CAD build for the part. Positions are in the model's coordinates, mm. A direction names the side the tool comes from. Round coordinates to 2 decimals unless told otherwise and drop trailing zeros. Write each loop counter-clockwise with the first axis right and the second up, starting at its lowest first coordinate (ties: lowest second). Pieces come first, ordered by that corner, then holes. Notation, with made-up numbers: (23.25, 46.5) -> (66.25, 46.5) arc R19 ccw to (66.25, 74.5) -> close; hole circle Ø3 at (-31.5, -14). An arc over 180 degrees is marked (long way). Put each result on its own line as item: value. Start each with the question number.
1. 3-axis set-ups, long thin cutter, end or side, ignore diameter. For faces 4 (the cylindrical face through (5, -15, -28)), 5 (the flat face through (5, -18, -26)), 6 (the flat face through (1, -15, 29)): which of +Z, -Z, +X, -X, +Y, -Y reach the whole face in a straight line?
2. Flat gauge pins, fed straight in: P1, Ø3, axis at x = 3, y = -17, coming from the +Z side; P2, Ø4, axis at x = 5, z = 32.5, coming from the +Y side; P3, Ø0.7, axis at x = 8.5, y = -15.5, coming from the -Z side. Where does each tip first touch, or does it go through?
3. Drill centre lines: line 1 (Z direction, x = 5, y = -32.75); line 2 (Z direction, x = 0.75, y = -6.5); line 3 (X direction, y = -33.7, z = -32.5). Where is each one in solid material? Low to high. Write a range as from..to.
4. Saw through at D-D on z = 20.5. List the corners of the cut face in (x, y).
5. Saw through at C-C on x = 1. List the corners of the cut face in (y, z).
6. Saw through at A-A on x = 5. List the corners of the cut face in (y, z).
7. Pull direction Z, two halves, no side cores. Call faces 1 (the cylindrical face through (5, -15, 28)), 2 (the flat face through (4.9, -35, 30.6)), 3 (the cylindrical face through (5.07, -0.57, 25.4)): pulls with the +Z half, pulls with the -Z half, needs draft (parallel to the pull), parting line crosses it, or undercut.
8. Saw through at B-B on z = 32.5. List the corners of the cut face in (x, y).
Autodesk Inventor part; units mm, degrees
ref_plane "YZ Plane" through (0, 0, 0) normal (1, 0, 0) x (0, 1, 0)
ref_plane "XZ Plane" through (0, 0, 0) normal (0, 1, 0) x (-1, 0, 0)
ref_plane "XY Plane" through (0, 0, 0) normal (0, 0, 1) x (1, 0, 0)
sketch "Sketch1" plane through (0, 0, 0) normal (1, 0, 0) x (0, 1, 0)
  line L0 (0, 0) -> (0, 26)
  line L1 (0, 26) -> (-35, 26)
  line L2 (0, 0) -> (3, 0)
  line L3 (3, 0) -> (3, 29)
  line L4 (3, 29) -> (-32, 29)
  line L5 (-32, 29) -> (-32, 36)
  line L6 (-32, 36) -> (-35, 36)
  line L7 (-35, 36) -> (-35, 26)
  line L8 (0, 0) -> (0, -26)
  line L9 (0, -26) -> (-35, -26)
  line L10 (3, 0) -> (3, -29)
  line L11 (3, -29) -> (-32, -29)
  line L12 (-32, -29) -> (-32, -36)
  line L13 (-32, -36) -> (-35, -36)
  line L14 (-35, -36) -> (-35, -26)
  dimension "d0" = 26
  dimension "d1" = 35
  dimension "d2" = 3
  dimension "d3" = 29
  dimension "d4" = 35
  dimension "d5" = 7
extrude "Extrusion1" add sketch "Sketch1" along normal blind 10
fillet "Fillet1" radius 2 4 edges at (5, 3, 29) (5, 0, 26) (5, 0, -26) (5, 3, -29)
sketch "Sketch2" plane through (0, -32, 36) normal (0, 1, 0) x (1, 0, 0)
  line L0 (0, 7) -> (0, 0)
  line L1 (0, 3.5) -> (5, 3.5)
  line L2 (0, 62) -> (0, 72)
  line L3 (0, 72) -> (0, 68.5)
  line L4 (0, 68.5) -> (5, 68.5)
  point P0 (0, 36)
  dimension "d9" = 3.5
hole "Hole1" at (5, -32, 32.5) at (5, -32, -32.5) direction (0, -1, 0) diameter 3.4 end through all
sketch "Sketch3" plane through (0, -32, 36) normal (0, 1, 0) x (1, 0, 0)
  circle A0 centre (5, 3.5) radius 1.7
  circle A1 centre (5, 3.5) radius 4.5
  circle A2 centre (5, 68.5) radius 1.7
  circle A3 centre (5, 68.5) radius 4.5
  point P0 (0, 36)
  dimension "d17" = 9
  dimension "d18" = 9
extrude "Extrusion2" cut sketch "Sketch3" along normal through all
sketch "Sketch4" plane through (0, -35, 36) normal (0, 0, 1) x (1, 0, 0)
  line L0 (0, 3) -> (2.1716, 3)
  line L1 (0, 0) -> (10, 0)
  line L2 (0, 3) -> (10, 3)
  line L3 (10, 3) -> (10, 0)
  line L4 (10, 0) -> (0, 0)
  line L5 (0, 0) -> (0, 3)
  point P0 (0, 35)
extrude "Extrusion3" add sketch "Sketch4" along normal blind 2
sketch "Sketch5" plane through (0, -35, -36) normal (0, 0, -1) x (-1, 0, 0)
  line L0 (0, 0) -> (-10, 0)
  line L1 (0, 3) -> (-10, 3)
  line L2 (-10, 3) -> (-10, 0)
  line L3 (-10, 0) -> (0, 0)
  line L4 (0, 0) -> (0, 3)
  point P0 (0, 35)
extrude "Extrusion4" add sketch "Sketch5" along normal blind 2
properties part number "battery-bracket"
Return value:
1. face 4: -Z, +Y
1. face 5: +X, -X, -Y
1. face 6: +Z, +X, -X, +Y
2. P1: stops at z = 29
2. P2: stops at y = -32
2. P3: stops at z = -29
3. line 1: z = -38..-34.2, -30.8..-26, 26..30.8, 34.2..38
3. line 2: z = -29..-26, 26..29
3. line 3: x = 0..3.3, 6.7..10
4. outline: (0, 0) -> (10, 0) -> (10, 3) -> (0, 3) -> close
5. outline: (-35, -38) -> (-32, -38) -> (-32, -29) -> (1, -29) arc R2 ccw to (3, -27) -> (3, 27) arc R2 ccw to (1, 29) -> (-32, 29) -> (-32, 38) -> (-35, 38) -> (-35, 26) -> (-2, 26) arc R2 cw to (0, 24) -> (0, -24) arc R2 cw to (-2, -26) -> (-35, -26) -> close
6. outline: (-35, -38) -> (-32, -38) -> (-32, -34.2) -> (-35, -34.2) -> close; (-35, -30.8) -> (-32, -30.8) -> (-32, -28) -> (2.73, -28) arc R2 ccw to (3, -27) -> (3, 27) arc R2 ccw to (2.73, 28) -> (-32, 28) -> (-32, 30.8) -> (-35, 30.8) -> (-35, 26) -> (-2, 26) arc R2 cw to (0, 24) -> (0, -24) arc R2 cw to (-2, -26) -> (-35, -26) -> close; (-35, 34.2) -> (-32, 34.2) -> (-32, 38) -> (-35, 38) -> close
7. face 1: pulls with the +Z half
7. face 2: needs draft
7. face 3: undercut
8. outline: (0, -35) -> (3.3, -35) -> (3.3, -32) -> (0, -32) -> close; (6.7, -35) -> (10, -35) -> (10, -32) -> (6.7, -32) -> close
